Read the model definition and answer for the solid it produces. Units are mm, in the model's axes. Face numbers are marked on the shaded views. A direction names the side the tool comes from. Give positions to 0.01 mm unless a question says otherwise; leave off trailing zeros. Order: outer loops, then holes, each group sorted by start corner. A loop starts at its lowest first (then second) coordinate and runs counter-clockwise, first axis right, second up. Notation, with made-up numbers: (58, -36.5) - (70, -36.5) arc R20 ccw to (70, -24.5) - close; hole circle Ø8 at (-21.75, -34). An arc over 180 degrees is marked (long way). Return JSON: item names as keys, results as strings.
```python
from build123d import *

# Parameters (mm, degrees)
BOSS_EXTRUDE1_DEPTH            = 20
SKETCH2_W                      = 20
SKETCH2_H                      = 23.5
BOSS_EXTRUDE2_DEPTH            = 4.5
CUT_EXTRUDE1_DEPTH             = 15
SKETCH4_W                      = 20
SKETCH4_H                      = 28
BOSS_EXTRUDE3_DEPTH            = 4.5
F_6_3_6_3_DIAMETER_HOLE1_D     = 6.3
F_6_3_6_3_DIAMETER_HOLE1_DEPTH = 28
F_6_3_6_3_DIAMETER_HOLE2_D     = 6.3
FILLET2_START                  = -11
FILLET2_DEPTH                  = 22


with BuildPart() as part:
    # Sketch1 → Boss-Extrude1 (new body)
    with BuildSketch(Plane(origin=(-10, 0, 0), x_dir=(0, -1, 0), z_dir=(-1, 0, 0))):
        with BuildLine():
            Line((-28, 4.5), (-4.5, 4.5))
            Line((-4.5, 4.5), (-4.5, 28))
            Line((-4.5, 28), (-4.792893219, 27.707106781))
            add(Edge.make_bspline(
                [(-4.792893219, 27.707106781), (-12.430964406, 20.069035594), (-20.069035594, 12.430964406), (-27.707106781, 4.792893219)],
                knots=[0, 0, 0, 0, 1, 1, 1, 1], degree=3))
            Line((-27.707106781, 4.792893219), (-28, 4.5))
        make_face()
    extrude(amount=-BOSS_EXTRUDE1_DEPTH)

    # Sketch2 → Boss-Extrude2 (add)
    with BuildSketch(Plane.XZ.offset(-4.5)):
        with Locations((0, 16.25)):
            Rectangle(SKETCH2_W, SKETCH2_H)
    extrude(amount=BOSS_EXTRUDE2_DEPTH)

    # Sketch3 → Cut-Extrude1 (cut)
    with BuildSketch(Plane(origin=(-7.5, 0, 0), x_dir=(0, -1, 0), z_dir=(-1, 0, 0))):
        with BuildLine():
            Line((-4.5, 4.5), (-4.5, 28))
            Line((-4.5, 28), (-4.792893219, 27.707106781))
            add(Edge.make_bspline(
                [(-4.792893219, 27.707106781), (-12.430964406, 20.069035594), (-20.069035594, 12.430964406), (-27.707106781, 4.792893219)],
                knots=[0, 0, 0, 0, 1, 1, 1, 1], degree=3))
            Line((-27.707106781, 4.792893219), (-28, 4.5))
            Line((-28, 4.5), (-4.5, 4.5))
        make_face()
    extrude(amount=-CUT_EXTRUDE1_DEPTH, mode=Mode.SUBTRACT)

    # Sketch4 → Boss-Extrude3 (add)
    with BuildSketch(Plane(origin=(0, 0, 4.5), x_dir=(-1, 0, 0), z_dir=(0, 0, -1))):
        with Locations((0, 14)):
            Rectangle(SKETCH4_W, SKETCH4_H)
    extrude(amount=BOSS_EXTRUDE3_DEPTH)

    # Ø6.3 (6.3) Diameter Hole1
    with Locations(Plane(origin=(0, 0, 0), x_dir=(-1, 0, 0), z_dir=(0, 0, -1))):
        with Locations((0, 20)):
            Hole(F_6_3_6_3_DIAMETER_HOLE1_D / 2, depth=F_6_3_6_3_DIAMETER_HOLE1_DEPTH)

    # Ø6.3 (6.3) Diameter Hole2 (through all)
    with Locations(Plane(origin=(0, 4.5, 0), x_dir=(1, 0, 0), z_dir=(0, 1, 0))):
        with Locations((0, -20)):
            Hole(F_6_3_6_3_DIAMETER_HOLE2_D / 2)

    # Fillet2: read off the stored shape, not the designer's step
    # Fillet2 outline → Fillet2 (cut)
    with BuildSketch(Plane.YZ.offset(FILLET2_START)):
        with BuildLine():
            Line((28, 4.085786438), (28, 4.5))
            Line((28, 4.5), (27.707106781, 4.792893219))
            ThreePointArc((27.707106781, 4.792893219), (27.923879533, 4.46846987), (28, 4.085786438))
        make_face()
        with BuildLine():
            Line((4.792893219, 27.707106781), (4.5, 28))
            Line((4.5, 28), (4.085786438, 28))
            ThreePointArc((4.085786438, 28), (4.46846987, 27.923879533), (4.792893219, 27.707106781))
        make_face()
    extrude(amount=FILLET2_DEPTH, mode=Mode.SUBTRACT)


solid = part.part
```
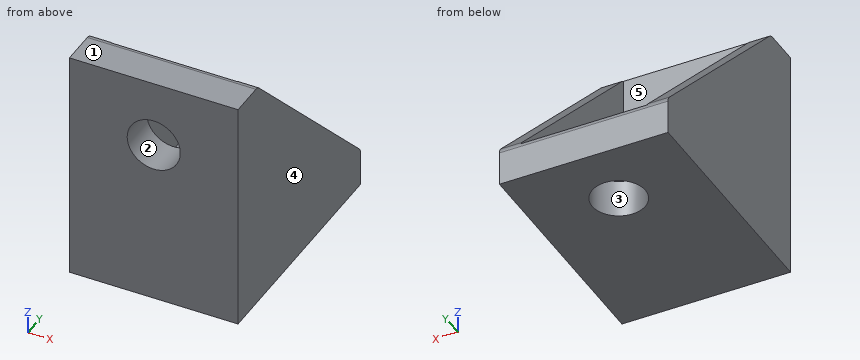
Q1. A cutting plane is placed at D-D (z = 25.75). Write down the section's boundary in (x, y).
Values:
{"outline": "(-10, 0) - (10, 0) - (10, 6.75) - (7.5, 6.75) - (7.5, 4.5) - (-7.5, 4.5) - (-7.5, 6.75) - (-10, 6.75) - close"}
Q2. A cutting plane is placed at C-C (y = 18). Write down the section's boundary in (x, z).
Values:
{"outline": "(-10, 0) - (-2.43, 0) - (-2.43, 4.5) - (-7.5, 4.5) - (-7.5, 14.5) - (-10, 14.5) - close; (2.43, 0) - (10, 0) - (10, 14.5) - (7.5, 14.5) - (7.5, 4.5) - (2.43, 4.5) - close"}
Q3. Determine the mould class of the marked faces 1, 2 and 3 for opening direction Z: released by +Z, released by -Z, zero draft, split by the parting line, or undercut.
Values:
{"face 1": "released by +Z", "face 2": "undercut", "face 3": "zero draft"}
Q4. Consider L1, parallel to Z at x = 0, y = 1.25; L2, parallel to X at y = 2.35, z = 20; L3, parallel to X at y = 5, z = 23. Determine where each line is inside the solid, lowest interval first.
Values:
{"L1": "z = 0 to 16.85, 23.15 to 28", "L2": "x = -10 to -3.15, 3.15 to 10", "L3": "x = -10 to -7.5, 7.5 to 10"}
Q5. Given pin 1 (3 mm diameter, centred on x = 7.5, z = 6, fed in from +Y); pin 2 (1 mm diameter, centred on x = 1, z = 7, fed in from +Y); pin 3 (5.5 mm diameter, centred on x = 0, y = 20, fed in from +Z); pin 4 (7.5 mm diameter, centred on x = -2, y = 21, fed in from +Z), each flat-ended and moving along its own axis, determine where each tip first touches the part or whether it passes through.
Values:
{"pin 1": "stops at y = 27.91", "pin 2": "stops at y = 4.5", "pin 3": "passes through", "pin 4": "stops at z = 4.5"}
Q6. A cutting plane is placed at A-A (x = 0). Write down the section's boundary in (y, z).
Values:
{"outline": "(0, 0) - (16.85, 0) - (16.85, 4.5) - (4.5, 4.5) - (4.5, 16.85) - (0, 16.85) - close; (0, 23.15) - (4.5, 23.15) - (4.5, 27.91) arc R1 ccw to (4.09, 28) - (0, 28) - close; (23.15, 0) - (28, 0) - (28, 4.09) arc R1 ccw to (27.91, 4.5) - (23.15, 4.5) - close"}
Q7. A cutting plane is placed at B-B (z = 20). Write down the section's boundary in (x, y), and give its area (3 significant figures).
Values:
{"outline": "(-10, 0) - (-3.15, 0) - (-3.15, 4.5) - (-7.5, 4.5) - (-7.5, 12.5) - (-10, 12.5) - close; (3.15, 0) - (10, 0) - (10, 12.5) - (7.5, 12.5) - (7.5, 4.5) - (3.15, 4.5) - close", "area": "102 mm²"}
Q8. For the marked faces 4 and 5, determine the directions among +Z, -Z, +X, -X, +Y, -Y from which every point of the face is accessible in a straight line to the end or side of a thin tool.
Values:
{"face 4": "+Z, -Z, +X, +Y, -Y", "face 5": "+Z, +Y"}
